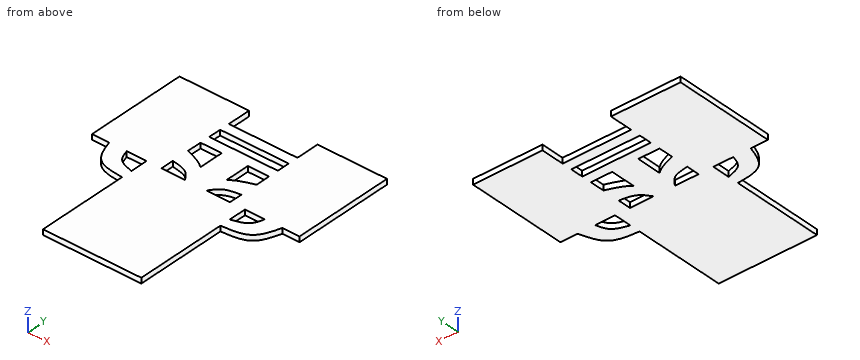
from build123d import *

# Parameters (mm, degrees)
F0_W     = 40.7416
F0_H     = 5.9913918376
F1_DEPTH = 3.175


# Not quite as in the source:
# - a feature names something its author has since deleted; it is built from what else it names


with BuildPart() as f1:
    # F0 (on Top) → F1 (new body)
    with BuildSketch(Plane.XY):
        Polygon((6.35, 2.420714612), (0, 2.420714612), (-6.35, 2.420714612), (-20.3708, 2.420714612), (-22.9107162118, 2.420714612), (-29.21, 2.420714612), (-29.21, -8.0478828564), (-29.21, -14.3978828564), (-29.21, -68.699285388), (29.21, -68.699285388), (29.21, -14.3978828564), (29.21, -8.0478828564), (29.21, 2.420714612), (20.3708, 2.420714612), align=None)
        Polygon((20.3708, 10.1967882365), (20.3708, 2.420714612), (29.21, 2.420714612), (41.0083, 2.420714612), (51.4477, 2.420714612), (61.6458, 2.420714612), (61.6458, 62.491714612), (20.3708, 62.491714612), (20.3708, 48.6805066466), (20.3708, 42.689114809), (20.3708, 35.2035965675), (20.3708, 29.2091965675), (20.3708, 20.6410996616), align=None)
        Polygon((-22.9107162118, 2.420714612), (-20.3708, 2.420714612), (-20.3708, 10.1967882365), (-20.3708, 20.6410996616), (-20.3708, 29.2091965675), (-20.3708, 35.2035965675), (-20.3708, 42.689114809), (-20.3708, 48.6805066466), (-20.3708, 62.491714612), (-61.6458, 62.491714612), (-61.6458, 2.420714612), (-51.4477, 2.420714612), (-41.0083, 2.420714612), (-29.21, 2.420714612), align=None)
        with BuildLine():
            add(Edge.make_bspline(
                [(29.21, -8.0478828564), (32.5638420451, -7.1347003919), (38.8822247108, -5.4143342635), (40.3293289084, -0.0814412218), (41.0083, 2.420714612)],
                knots=[0, 0, 0, 0, 0.5308070471, 1, 1, 1, 1], degree=3))
            Line((29.21, -8.0478828564), (29.21, -14.3978828564))
            add(Edge.make_bspline(
                [(29.21, -14.3978828564), (35.0623442189, -14.0006727781), (46.562333527, -13.2201459527), (49.8386841247, -2.7306682151), (51.4477, 2.420714612)],
                knots=[0, 0, 0, 0, 0.5088999704, 1, 1, 1, 1], degree=3))
            Line((51.4477, 2.420714612), (41.0083, 2.420714612))
        make_face()
        with BuildLine():
            Line((-29.21, -14.3978828564), (-29.21, -8.0478828564))
            add(Edge.make_bspline(
                [(-29.21, -8.0478828564), (-32.5638420451, -7.1347003919), (-38.8822247108, -5.4143342635), (-40.3293289084, -0.0814412218), (-41.0083, 2.420714612)],
                knots=[0, 0, 0, 0, 0.5308070471, 1, 1, 1, 1], degree=3))
            Line((-41.0083, 2.420714612), (-51.4477, 2.420714612))
            add(Edge.make_bspline(
                [(-29.21, -14.3978828564), (-35.0623442189, -14.0006727781), (-46.562333527, -13.2201459527), (-49.8386841247, -2.7306682151), (-51.4477, 2.420714612)],
                knots=[0, 0, 0, 0, 0.5088999704, 1, 1, 1, 1], degree=3))
        make_face()
        with Locations((0, 45.6848107278)):
            Rectangle(F0_W, F0_H)
        with BuildLine():
            Line((-6.35, 2.420714612), (0, 2.420714612))
            add(Edge.make_bspline(
                [(0, 2.420714612), (-2.1599363926, 6.9765171348), (-4.3198727852, 11.5323196577), (-7.7523121432, 14.5766604692)],
                knots=[0, 0, 0, 0, 0.5036722623, 0.5036722623, 0.5036722623, 0.5036722623], degree=3))
            add(Edge.make_bspline(
                [(-7.7523121432, 14.5766604692), (-11.1346998365, 17.5766088502), (-15.7527499182, 19.1088542559), (-20.3708, 20.6410996616)],
                knots=[0.5036722623, 0.5036722623, 0.5036722623, 0.5036722623, 1, 1, 1, 1], degree=3))
            Line((-20.3708, 20.6410996616), (-20.3708, 10.1967882365))
            add(Edge.make_bspline(
                [(-6.35, 2.420714612), (-7.7523121432, 4.4872624945), (-10.7420432518, 8.8931449662), (-17.0314139567, 9.7446667159), (-20.3708, 10.1967882365)],
                knots=[0, 0, 0, 0, 0.4690428979, 1, 1, 1, 1], degree=3))
        make_face()
        with BuildLine():
            add(Edge.make_bspline(
                [(0, 2.420714612), (2.1599363926, 6.9765171348), (4.3198727852, 11.5323196577), (7.7523121432, 14.5766604692)],
                knots=[0, 0, 0, 0, 0.5036722623, 0.5036722623, 0.5036722623, 0.5036722623], degree=3))
            Line((0, 2.420714612), (6.35, 2.420714612))
            add(Edge.make_bspline(
                [(6.35, 2.420714612), (7.7523121432, 4.4872624945), (10.7420432518, 8.8931449662), (17.0314139567, 9.7446667159), (20.3708, 10.1967882365)],
                knots=[0, 0, 0, 0, 0.4690428979, 1, 1, 1, 1], degree=3))
            Line((20.3708, 10.1967882365), (20.3708, 20.6410996616))
            add(Edge.make_bspline(
                [(7.7523121432, 14.5766604692), (11.1346998365, 17.5766088502), (15.7527499182, 19.1088542559), (20.3708, 20.6410996616)],
                knots=[0.5036722623, 0.5036722623, 0.5036722623, 0.5036722623, 1, 1, 1, 1], degree=3))
        make_face()
        with BuildLine():
            add(Edge.make_bspline(
                [(0, 2.420714612), (-2.1599363926, 6.9765171348), (-4.3198727852, 11.5323196577), (-7.7523121432, 14.5766604692)],
                knots=[0, 0, 0, 0, 0.5036722623, 0.5036722623, 0.5036722623, 0.5036722623], degree=3))
            add(Edge.make_bspline(
                [(0, 2.420714612), (2.1599363926, 6.9765171348), (4.3198727852, 11.5323196577), (7.7523121432, 14.5766604692)],
                knots=[0, 0, 0, 0, 0.5036722623, 0.5036722623, 0.5036722623, 0.5036722623], degree=3))
            Line((7.7523121432, 14.5766604692), (7.7523121432, 29.2091965675))
            Line((7.7523121432, 29.2091965675), (-7.7523121432, 29.2091965675))
            Line((-7.7523121432, 29.2091965675), (-7.7523121432, 14.5766604692))
        make_face()
        Polygon((-7.7523121432, 29.2091965675), (7.7523121432, 29.2091965675), (20.3708, 29.2091965675), (20.3708, 35.2035965675), (-20.3708, 35.2035965675), (-20.3708, 29.2091965675), align=None)
    extrude(amount=F1_DEPTH)


solid = f1.part
Geometry: final body of the model. Coordinates: model frame, mm. Give positions to 0.01 mm unless a question says otherwise; leave off trailing zeros. Loops run counter-clockwise (first coordinate to the right, second up) from the corner with the lowest first, then second, coordinate; pieces in that order, holes last. Notation, with made-up numbers: (50.25, -3.5) - (70.25, -3.5) arc R34 ccw to (70.25, 30.5) - close; hole circle Ø9 at (89, 27). An arc over 180 degrees is marked (long way). One line per question, with ' | ' between items. Start each with the question number.
(1) Section query B-B on z = 2.55. Count the separate pieces of the cut face and the enclosed holes in it, then the cut area to 3 significant figures.
(2) Ray query, line 1 (X direction, y = 22, z = 1.6); line 2 (X direction, y = 41, z = 2.65); line 3 (Y direction, x = 1, z = 1.55). Return the intervals inside material, ascending. Write a range as from..to.
(3) Section query D-D on y = -49. Return loops of the section in (x, z) (3 decimals), then the cut area to 3 significant figures.
(4) Section query A-A on x = 1.5. Return loops of the section in (y, z) (1 decimal), then the cut area to 3 significant figures.
(5) Contact query for flat-ended pins moving along their axis: pin 1 (1 mm diameter, centred on y = -44.5, z = 1.5, fed in from -X); pin 2 (1 mm diameter, centred on x = -3.5, z = 2, fed in from +Y); pin 3 (1 mm diameter, centred on y = -5.5, z = 2, fed in from +X). Output: stop coordinate, or through.
The answers:
1) separate pieces: 1 | enclosed holes: 7 | area: 10,700 mm2
2) line 1: -61.65..-20.37, -7.75..7.75, 20.37..61.65 | line 2: -61.65..-20.37, 20.37..61.65 | line 3: -68.7..35.2, 42.69..48.68
3) outline: (-29.21, 0) - (29.21, 0) - (29.21, 3.175) - (-29.21, 3.175) - close | area: 185 mm2
4) outline: (-68.7, 0) - (35.2, 0) - (35.2, 3.2) - (-68.7, 3.2) - close; (42.7, 0) - (48.7, 0) - (48.7, 3.2) - (42.7, 3.2) - close | area: 349 mm2
5) pin 1: x = -29.21 | pin 2: y = 48.68 | pin 3: x = 48.79
